Job drawing, mm, ordinate dimensions from the low corner. One solid piece. A direction names the side the tool comes from. Coordinates: 2 decimals unless noted, no trailing zeros. Loops run counter-clockwise (first coordinate to the right, second up) from the corner with the lowest first, then second, coordinate; pieces in that order, holes last. Notation, with made-up numbers: (54.25, 44) -> (103.25, 44) arc R29 cw to (103.25, 70) -> close; hole circle Ø9 at (45.25, 56). An arc over 180 degrees is marked (long way). Use one line per item in the form item = value. Start each with the question number.
(1) Band-saw the part on B-B on z = 9. Give the cut face in (x, y).
(2) Drill centre lines: L1, parallel to Y at x = 23, z = 17.5; L2, parallel to Z at x = 15, y = 63.5; L3, parallel to X at y = 81, z = 41. Where is each one in solid material? Low to high. Write a range as [from, to].
(3) 3-axis set-ups, long thin cutter, end or side, ignore diameter. For the marked faces 1, 2 and 3: which of +Z, -Z, +X, -X, +Y, -Y reach the whole face in a straight line?
(4) Band-saw the part on C-C on y = 36. Give the cut face in (x, z).
(5) Band-saw the part on A-A on x = 15.5. Give the cut face in (y, z).
(6) Band-saw the part on D-D on y = 67. Give the cut face in (x, z), then the cut area to 3 significant figures.
(7) Pin check, flat tips, straight feed: P1, Ø22, axis at x = 7, y = 57.5, coming from the -Z side; P2, Ø16, axis at x = 8, z = 9.5, coming from the +Y side; P3, Ø2, axis at y = 38.5, z = 23, coming from the +X side; P4, Ø12, axis at x = 7.5, z = 6.5, coming from the -Y side. Stop position of each tip, or through.
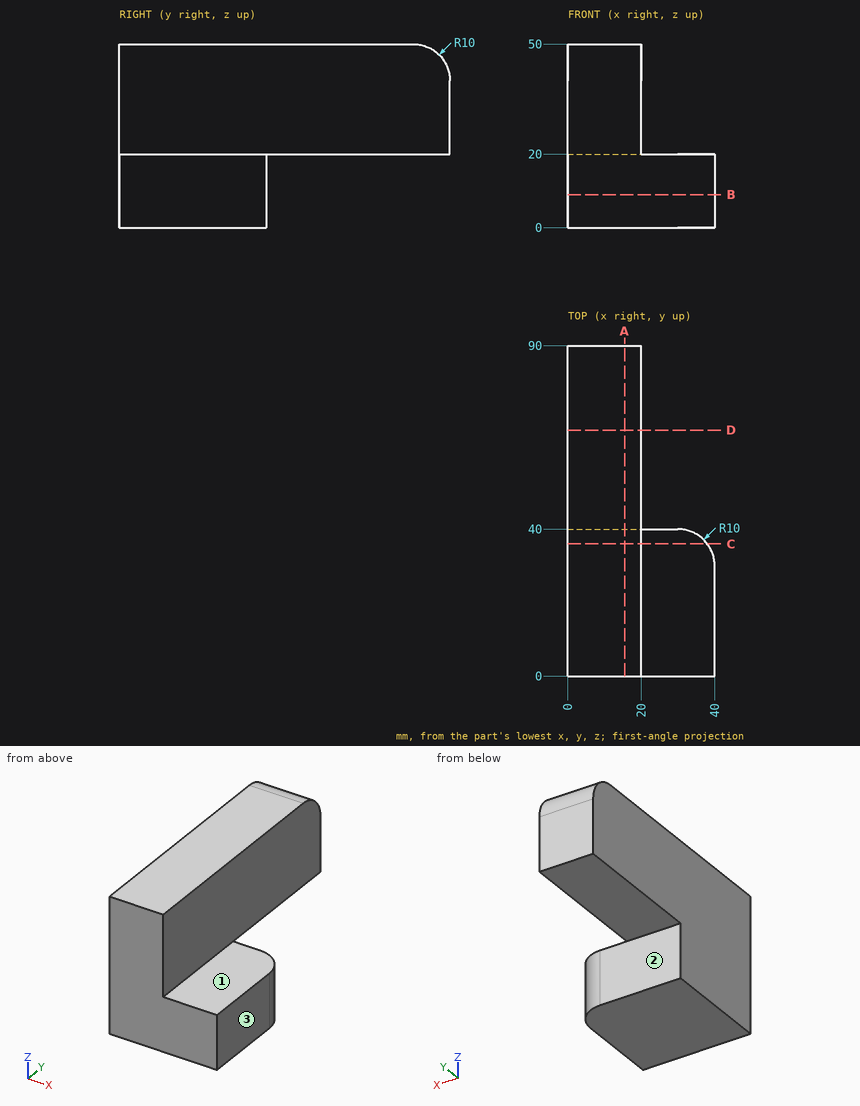
A:
q1.outline = (0, 0) -> (40, 0) -> (40, 30) arc R10 ccw to (30, 40) -> (0, 40) -> close
q2.L1 = [0, 40]
q2.L2 = [20, 50]
q2.L3 = [0, 20]
q3.face_1 = +Z, +X, +Y, -Y
q3.face_2 = -Z, +X, -X, +Y
q3.face_3 = +Z, -Z, +X, +Y, -Y
q4.outline = (0, 0) -> (38, 0) -> (38, 20) -> (20, 20) -> (20, 50) -> (0, 50) -> close
q5.outline = (0, 0) -> (40, 0) -> (40, 20) -> (90, 20) -> (90, 40) arc R10 ccw to (80, 50) -> (0, 50) -> close
q6.outline = (0, 20) -> (20, 20) -> (20, 50) -> (0, 50) -> close
q6.area = 600 mm²
q7.P1 = 20
q7.P2 = 40
q7.P3 = 20
q7.P4 = 0
